from build123d import *

# Parameters (mm, degrees)
SKETCH1_R           = 2.5
SKETCH1_R_2         = 2.25
BOSS_EXTRUDE1_DEPTH = 4


with BuildPart() as part:
    # Sketch1 → Boss-Extrude1 (new body)
    with BuildSketch(Plane(origin=(0, 0, 0), x_dir=(1, 0, 0), z_dir=(0, 1, 0))):
        with BuildLine():
            Line((1.764581835, 8.584003487), (0, 8.763496159))
            ThreePointArc((0, 8.763496159), (-8.763496159, 0), (0, -8.763496159))
            Line((0, -8.763496159), (76.322471515, -11))
            Line((76.322471515, -11), (76.322471515, 1))
            Line((76.322471515, 1), (1.764581835, 8.584003487))
        make_face()
        with Locations((70.322471515, -5)):
            Circle(SKETCH1_R, mode=Mode.SUBTRACT)
        Circle(SKETCH1_R_2, mode=Mode.SUBTRACT)
    extrude(amount=BOSS_EXTRUDE1_DEPTH)


solid = part.part
Read the model definition and answer for the solid it produces. Units are mm, in the model's axes. Round coordinates to 2 decimals unless told otherwise and drop trailing zeros. Write each loop counter-clockwise with the first axis right and the second up, starting at its lowest first coordinate (ties: lowest second). Pieces come first, ordered by that corner, then holes.
1. Determine the mould class of faces 1 (the face through (33, 0, 1)), 2 (the face through (-0.29, 1.97, -2.23)), 3 (the face through (76.322, 2, 5)) for opening direction X: pulls with the +X half, pulls with the -X half, needs draft (parallel to the pull), parting line crosses it, or undercut.
2. The part is cut by section A-A, the plane z = 0. Determine the outline of the cut face in (x, y).
3. The part is cut by section C-C, the plane z = 6. Determine the outline of the cut face in (x, y).
4. The part is cut by section D-D, the plane x = 60. Determine the outline of the cut face in (y, z).
5. Straight lines are drawn through the part: L1, parallel to X at y = 2.2, z = 0; L2, parallel to X at y = 1.4, z = 5.5; L3, parallel to Z at x = -4.5, y = 2.55. For each, find the intervals that lie inside material, in ascending order.
6. Given pin 1 Ø2 at (y, z) = (2, 2.5) entering from -X; pin 2 Ø1 at (x, y) = (12.5, 2.5) entering from +Z, each flat-ended and moving along its own axis, determine where each tip first touches the part or whether it passes through.
7. The part is cut by section B-B, the plane y = 0.9. Determine the outline of the cut face in (x, z), then the cut area to 3 significant figures.
Values:
1. face 1: needs draft
1. face 2: undercut
1. face 3: pulls with the +X half
2. outline: (-8.76, 0) - (-2.25, 0) - (-2.25, 4) - (-8.76, 4) - close; (2.25, 0) - (76.32, 0) - (76.32, 4) - (2.25, 4) - close
3. outline: (-6.39, 0) - (68.03, 0) - (68.03, 4) - (-6.39, 4) - close; (72.61, 0) - (76.32, 0) - (76.32, 4) - (72.61, 4) - close
4. outline: (0, -2.66) - (4, -2.66) - (4, 10.52) - (0, 10.52) - close
5. L1: x = -8.76 to -2.25, 2.25 to 76.32
5. L2: x = -6.82 to 67.87, 72.77 to 76.32
5. L3: z = -7.52 to 7.52
6. pin 1: stops at x = -8.63
6. pin 2: stops at z = 9.14
7. outline: (0, -8.76) - (76.32, -1) - (76.32, 11) - (0, 8.76) arc R8.76 ccw to start; hole circle Ø4.5 at (0, 0); hole circle Ø5 at (70.32, 5)
7. area: 1,210 mm2
